Can you work these out from the drawing? Everything is in mm from the part's minimum corner. A direction names the side the tool comes from. Round coordinates to 2 decimals unless told otherwise and drop trailing zeros. Order: outer loops, then holes, each group sorted by start corner. A loop starts at its lowest first (then second) coordinate and runs counter-clockwise, first axis right, second up. Notation, with made-up numbers: M 74,8 L 115,8 A31 cw 115,47 Z; hole C 14,71 d2. An arc over 180 degrees is marked long. Write item = value, one per line. Start each with the question number.
Item 1: I'm going to push a flat-ended pin straight in: P1, Ø1.5, axis at x = 10, z = 21.5, coming from the -Y side. Where does the tip first touch, or does it pass through?
Item 2: For the marked faces 1 and 2, which set-ups out of +Z, -Z, +X, -X, +Y, -Y let a thin tool reach every point of the face, with its end or its side?
Item 3: I want a section at C-C, the plane x = 31. List the corners of the cut face in (y, z) for me, plus the area to 3 significant figures.
Item 4: I want a section at D-D, the plane x = 21. List the corners of the cut face in (y, z) for me.
Item 5: I want a section at B-B, the plane y = 31. List the corners of the cut face in (x, z) for me (1 decimal), plus the area to 3 significant figures.
Item 6: I want a section at A-A, the plane z = 25. List the corners of the cut face in (x, y) for me (1 decimal).
Item 7: Please list where these lines run through material, in increasing order: L1, parallel to Z at x = 33, y = 41.5; L2, parallel to Z at x = 36.5, y = 34 (1 decimal); L3, parallel to Y at x = 15, z = 9.
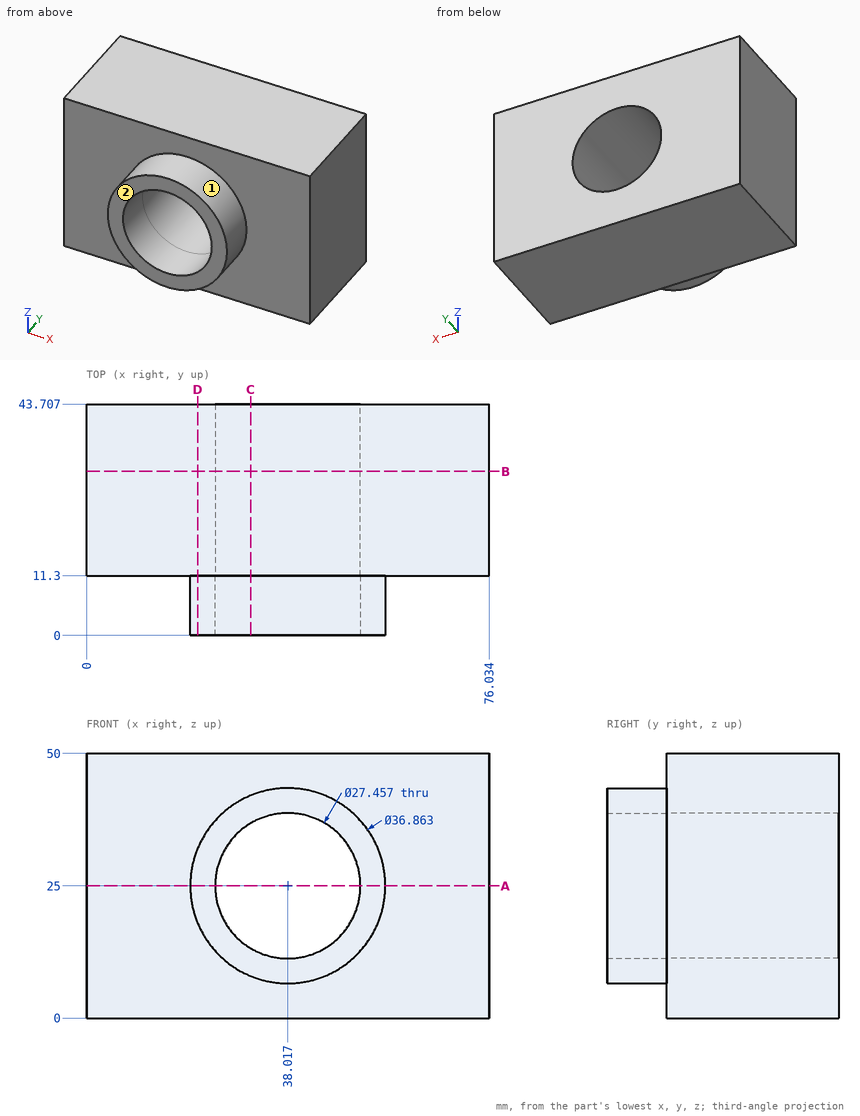
Filled in:
q1.P1 = 11.3
q2.face_1 = -Y
q2.face_2 = +Z, -Z, +X, -X, -Y
q3.outline = M 0,7.96 L 11.3,7.96 L 11.3,0 L 43.71,0 L 43.71,13.2 L 0,13.2 Z; M 0,36.8 L 43.71,36.8 L 43.71,50 L 11.3,50 L 11.3,42.04 L 0,42.04 Z
q3.area = 974 mm^2
q4.outline = M 0,17.92 L 11.3,17.92 L 11.3,0 L 43.71,0 L 43.71,50 L 11.3,50 L 11.3,32.08 L 0,32.08 Z
q5.outline = M 0,0 L 76,0 L 76,50 L 0,50 Z; hole C 38,25 d27.5
q5.area = 3,210 mm^2
q6.outline = M 0,11.3 L 19.6,11.3 L 19.6,0 L 24.3,0 L 24.3,43.7 L 0,43.7 Z; M 51.7,0 L 56.4,0 L 56.4,11.3 L 76,11.3 L 76,43.7 L 51.7,43.7 Z
q7.L1 = 0 to 12.22, 37.78 to 50
q7.L2 = 0 to 11.4, 38.6 to 50
q7.L3 = 11.3 to 43.71
